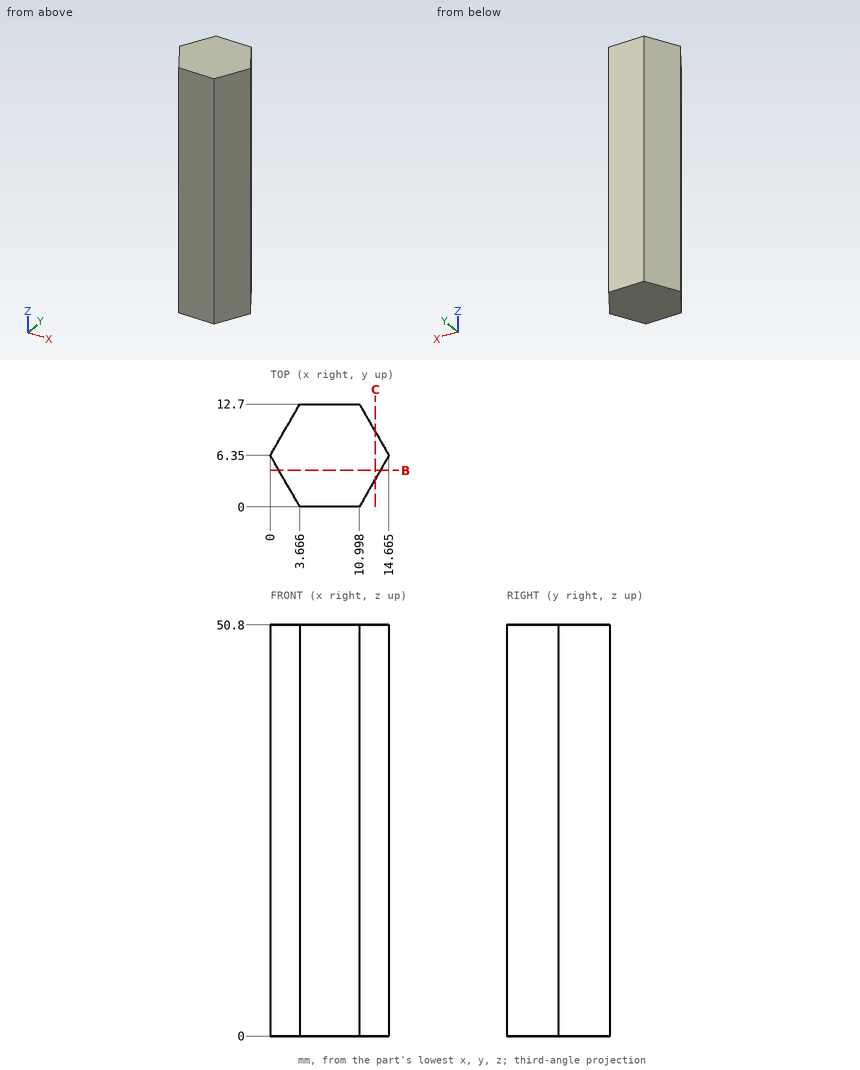
Design review of the part shown in the three views and the two pictorial views. Dimensions are in mm from the part's minimum x, y and z. Give positions to 0.01 mm unless a question says otherwise; leave off trailing zeros. Loops run counter-clockwise (first coordinate to the right, second up) from the corner with the lowest first, then second, coordinate; pieces in that order, holes last. Notation, with made-up numbers: M 38.25,30 L 96.25,30 A24 ccw 96.25,62 Z; hole C -19,57.25 d1. An arc over 180 degrees is marked long. Answer as a JSON object with one key per item and string values. Group by question number.
Q1. Add section C-C on x = 13. Give the boundary of the cut face in (y, z).
Q2. Insertion check: P1, Ø1.5, axis at y = 10.5, z = 42, coming from the -X side; P2, Ø1.5, axis at y = 3, z = 22, coming from the -X side; P3, Ø3, axis at y = 11, z = 5.5, coming from the -X side. Each pin has a flat end and moves straight along its axis. Give the tip position at first contact, or say it passes through.
Q3. Add section B-B on y = 4.5. Give the boundary of the cut face in (x, z).
Q4. For probe 1 along Y at (x, z) = (13.25, 40); probe 2 along X at (y, z) = (8, 5); probe 3 along X at (y, z) = (7.75, 47) (1 decimal), list the stretches that pass through material, from the lowest coordinate up. Write a range as [from, to].
Checked values:
{
 "1": {"outline": "M 3.47,0 L 9.23,0 L 9.23,50.8 L 3.47,50.8 Z"},
 "2": {"P1": "x = 1.96", "P2": "x = 1.5", "P3": "x = 1.82"},
 "3": {"outline": "M 1.07,0 L 13.6,0 L 13.6,50.8 L 1.07,50.8 Z"},
 "4": {"probe 1": "[3.9, 8.8]", "probe 2": "[0.95, 13.71]", "probe 3": "[0.8, 13.9]"}
}
